Can you work these out from the model? Positions are in its coordinate system, mm. A direction names the side the tool comes from. Coordinates: 2 decimals unless noted, no trailing zeros. Write each loop counter-clockwise with the first axis right and the second up, starting at its lowest first coordinate (ties: lowest second). Pieces come first, ordered by that corner, then holes. Notation, with made-up numbers: (22.5, -39) - (55.5, -39) arc R12 ccw to (55.5, -16) - close; hole circle Ø6 at (49.25, 21.25). An arc over 180 degrees is marked (long way). Use one line per item in the form item = value. Start each with the question number.
(1) On a 3-axis mill with a long thin cutter (end or side, diameter ignored), from which of +Z, -Z, +X, -X, +Y, -Y can I reach the whole of each face in a straight line? I mean faces 5 (the face through (52.85, 27.01, 4.93)), 6 (the face through (-52.85, 27.01, 4.93)), 7 (the face through (84, 7, 5)), 8 (the face through (31.6, 236, 5)), 9 (the face through (-31.6, 236, 5)). Say none if no direction works.
(2) If we section it at D-D on x = -42: Please give me the cut outline in (y, z).
(3) If I drill on probe 1 along X at (y, z) = (117.5, 3.75); probe 2 along Y at (x, z) = (0.5, 8.75); probe 3 along X at (y, z) = (60, 6.75), over which ranges is the centre line in solid material (lowest first)? Write a range as from..to.
(4) For pin 1 Ø3 at (y, z) = (61, 3) entering from -X; pin 2 Ø22.5 at (x, y) = (0, 117.5) entering from +Z; pin 3 Ø4 at (y, z) = (195, 7) entering from +X; pin 4 Ø2 at (y, z) = (116.5, 8.5) entering from +X, each with a flat end and sliding along its axis, tell me the tip position at first contact or that it passes through.
(5) Thinking about a two-plate mould opening in Y: for faces 1 (the face through (67, 24, 5)), 2 (the face through (-84, 7, 5)), 3 (the face through (-81.15, 20.99, 4.93)), 4 (the face through (50, 59, 5)), which applies, pulls with the +Y half, pulls with the -Y half, needs draft (parallel to the pull), parting line crosses it, or undercut?
(6) If we section it at B-B on z = 8: Give the number of separate pieces and of enclosed holes in the cut face, then the cut area to 3 significant figures.
(7) If we section it at C-C on y = 125: Please give me the cut outline in (x, z).
(8) If we section it at A-A on y = 60: Please give me the cut outline in (x, z), then the cut area to 3 significant figures.
```python
from build123d import *

# Parameters (mm, degrees)
PAD_DEPTH = 10


with BuildPart() as part:
    # Sketch → Pad (new body)
    with BuildSketch(Plane.XY):
        with BuildLine():
            Line((0, 0), (84, 0))
            Line((84, 0), (84, 14))
            ThreePointArc((84, 14), (81.071068, 21.071068), (74, 24))
            Line((60, 24), (74, 24))
            ThreePointArc((50, 34), (52.928932, 26.928932), (60, 24))
            Line((50, 34), (50, 84.033599))
            ThreePointArc((55.263158, 92.840547), (51.416049, 89.163491), (50, 84.033599))
            ThreePointArc((55.263158, 92.840547), (66.035062, 103.136303), (70, 117.5))
            ThreePointArc((70, 117.5), (64.624358, 144.40153), (49.323077, 167.17126))
            ThreePointArc((31.6, 209.746626), (36.207693, 186.688172), (49.323077, 167.17126))
            Line((31.6, 209.746626), (31.6, 263))
            ThreePointArc((31.6, 263), (22.344574, 285.344574), (0, 294.6))
            Line((0, 294.6), (0, 281.35))
            ThreePointArc((0, 244.65), (18.35, 263), (0, 281.35))
            Line((0, 244.65), (0, 173.5))
            ThreePointArc((56, 117.5), (39.59798, 157.09798), (0, 173.5))
            ThreePointArc((28, 117.5), (42, 103.5), (56, 117.5))
            ThreePointArc((28, 117.5), (19.79899, 137.29899), (0, 145.5))
            Line((0, 145.5), (0, 131.5))
            ThreePointArc((0, 103.5), (14, 117.5), (0, 131.5))
            Line((0, 103.5), (0, 88.6))
            ThreePointArc((0, 31.4), (28.6, 60), (0, 88.6))
            Line((0, 31.4), (0, 0))
        make_face()
    pad = extrude(amount=PAD_DEPTH)

    # Mirrored: Pad across Sketch V_Axis
    add(pad.mirror(Plane(origin=(0, 0, 0), x_dir=(0, 0, 1), z_dir=(1, 0, 0))))


solid = part.part
```
Reported:
q1.face_5 = +Z, -Z, +X
q1.face_6 = +Z, -Z, -X
q1.face_7 = +Z, -Z, +X, +Y, -Y
q1.face_8 = +Z, -Z, +X, +Y
q1.face_9 = +Z, -Z, -X, +Y
q2.outline = (0, 0) - (103.5, 0) - (103.5, 10) - (0, 10) - close; (154.54, 0) - (175.99, 0) - (175.99, 10) - (154.54, 10) - close
q3.probe_1 = -70..-56, -28..-14, 14..28, 56..70
q3.probe_2 = 0..31.4, 88.6..103.51, 131.49..145.5, 173.5..244.66, 281.34..294.6
q3.probe_3 = -50..-28.6, 28.6..50
q4.pin_1 = -50
q4.pin_2 = through
q4.pin_3 = 33.98
q4.pin_4 = 70
q5.face_1 = undercut
q5.face_2 = needs draft
q5.face_3 = pulls with the +Y half
q5.face_4 = undercut
q6.separate_pieces = 1
q6.enclosed_holes = 4
q6.area = 20,000 mm2
q7.outline = (-69.6, 0) - (-55.5, 0) - (-55.5, 10) - (-69.6, 10) - close; (-26.98, 0) - (-11.82, 0) - (-11.82, 10) - (-26.98, 10) - close; (11.82, 0) - (26.98, 0) - (26.98, 10) - (11.82, 10) - close; (55.5, 0) - (69.6, 0) - (69.6, 10) - (55.5, 10) - close
q8.outline = (-50, 0) - (-28.6, 0) - (-28.6, 10) - (-50, 10) - close; (28.6, 0) - (50, 0) - (50, 10) - (28.6, 10) - close
q8.area = 428 mm2
